Check sheet for the modelled part. Datum: model origin and axes. Units: mm. Face numbers are marked on the shaded views. Give positions to 0.01 mm unless a question says otherwise; leave off trailing zeros. Loops run counter-clockwise (first coordinate to the right, second up) from the corner with the lowest first, then second, coordinate; pieces in that order, holes last. Notation, with made-up numbers: M 87,-20.5 L 123,-20.5 A19 cw 123,4.5 Z; hole C 43,-32 d2. An arc over 180 degrees is marked long. Use one line per item in the form item = value.
from build123d import *

# Parameters (mm, degrees)
CYLINDER_R        = 4.75
CYLINDER_DEPTH    = 10
CYLINDER001_R     = 6.25
CYLINDER001_DEPTH = 0.7
CYLINDER002_R     = 8
CYLINDER002_DEPTH = 0.7


with BuildPart() as cylinder:
    # Cylinder → Cylinder (new body)
    with BuildSketch(Plane.XY.offset(-4)):
        Circle(CYLINDER_R)
    extrude(amount=CYLINDER_DEPTH)


with BuildPart() as cylinder001:
    # Cylinder001 → Cylinder001 (new body)
    with BuildSketch(Plane.XY):
        Circle(CYLINDER001_R)
    extrude(amount=CYLINDER001_DEPTH)


with BuildPart() as washer:
    # Cylinder002 → Cylinder002 (new body)
    with BuildSketch(Plane.XY.offset(0.7)):
        Circle(CYLINDER002_R)
    extrude(amount=CYLINDER002_DEPTH)

    # Fusion: union Cylinder001
    add(cylinder001.part)

    # Cut: cut Cylinder
    add(cylinder.part, mode=Mode.SUBTRACT)


solid = washer.part
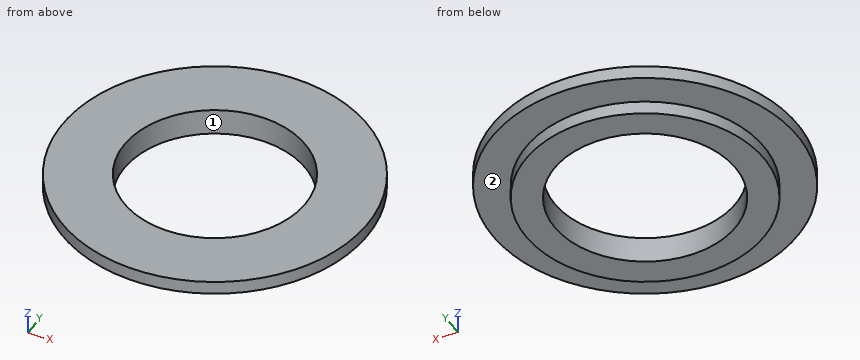
1) Section check A-A (y = 0). Record the cut outline in (x, z), then the cut area to 3 significant figures.
Evaluation:
outline = M -8,0.7 L -6.25,0.7 L -6.25,0 L -4.75,0 L -4.75,1.4 L -8,1.4 Z; M 4.75,0 L 6.25,0 L 6.25,0.7 L 8,0.7 L 8,1.4 L 4.75,1.4 Z
area = 6.65 mm^2
2) Section check C-C (z = 0.4). Record the cut outline in (x, y), then the cut area to 3 significant figures.
Evaluation:
outline = C 0,0 d12.5; hole C 0,0 d9.5
area = 51.8 mm^2
3) Section check D-D (y = 5.5). Record the cut outline in (x, z).
Evaluation:
outline = M -5.81,0.7 L -2.97,0.7 L -2.97,0 L 2.97,0 L 2.97,0.7 L 5.81,0.7 L 5.81,1.4 L -5.81,1.4 Z
4) Depth check by flat-ended pin: pin 1 Ø7.5 at (x, y) = (0, 0) entering from -Z; pin 2 Ø1.5 at (x, y) = (-5.5, -6) entering from -Z. Enter the tip coordinate at first touch or a pass-through.
Evaluation:
pin_1 = through
pin_2 = 0.7
5) Release check for a two-part mould opening along X. For the marked faces 1 and 2 record: pulls with the +X half, pulls with the -X half, needs draft (parallel to the pull), parting line crosses it, or undercut.
Evaluation:
face_1 = undercut
face_2 = needs draft
6) Scan lines: line 1 (Y direction, x = 0, z = 0.5); line 2 (Y direction, x = 0, z = 1.15); line 3 (Z direction, x = 5.75, y = -3). Record each from-to range of solid material in increasing order.
Evaluation:
line_1 = -6.25 to -4.75, 4.75 to 6.25
line_2 = -8 to -4.75, 4.75 to 8
line_3 = 0.7 to 1.4
